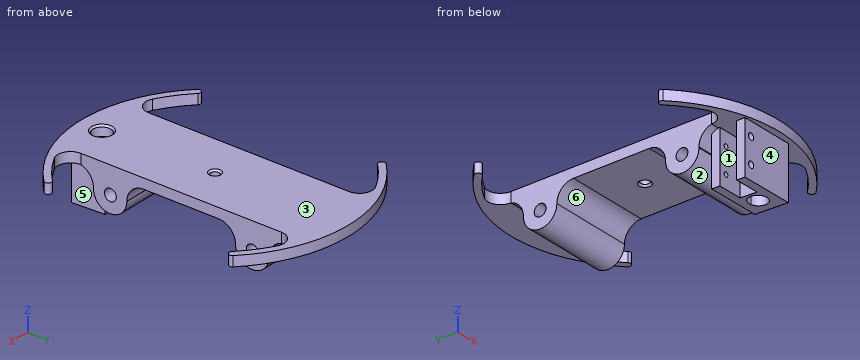
from build123d import *

# Parameters (mm, degrees)
BOSS_EXTRUDE2_DEPTH               = 3.81
BOSS_EXTRUDE4_DEPTH               = 31.75
F_8_CLEARANCE_HOLE1_D             = 4.4958
BOSS_EXTRUDE7_REACH               = 65.711
SKETCH19_R                        = 3.3782
F_1_4_CLEARANCE_HOLE3_D           = 6.7564
F_1_4_CLEARANCE_HOLE3_CSINK_D     = 8.0264
F_1_4_CLEARANCE_HOLE3_CSINK_ANGLE = 90
SKETCH25_R                        = 2.794
CUT_EXTRUDE1_DEPTH                = 3.81
F_2_CLEARANCE_HOLE1_D             = 2.4384
F_2_CLEARANCE_HOLE1_DEPTH         = 3.175
TAP_DRILL_FOR_2_56_TAP1_D         = 1.778
TAP_DRILL_FOR_2_56_TAP1_DEPTH     = 12.7


with BuildPart() as part:
    # Sketch3 → Boss-Extrude2 (new body)
    with BuildSketch(Plane.XY):
        with BuildLine():
            Line((-15.875, -38.1), (-15.875, 38.1))
            ThreePointArc((-15.875, 38.1), (-18.260491841, 42.291797068), (-23.082694008, 42.38179842))
            ThreePointArc((-23.082694008, 42.38179842), (-28.900226452, 38.649767283), (-34.12497326, 34.12497326))
            ThreePointArc((-34.12497326, 34.12497326), (-35.921024484, 34.12497326), (-35.921024484, 35.921024484))
            ThreePointArc((-35.921024484, 35.921024484), (0, 50.8), (35.921024484, 35.921024484))
            ThreePointArc((35.921024484, 35.921024484), (35.921024484, 34.12497326), (34.12497326, 34.12497326))
            ThreePointArc((34.12497326, 34.12497326), (28.900226452, 38.649767283), (23.082694008, 42.38179842))
            ThreePointArc((23.082694008, 42.38179842), (18.260491841, 42.291797068), (15.875, 38.1))
            Line((15.875, 38.1), (15.875, -38.1))
            ThreePointArc((15.875, -38.1), (18.260491841, -42.291797068), (23.082694008, -42.38179842))
            ThreePointArc((23.082694008, -42.38179842), (28.900226452, -38.649767283), (34.12497326, -34.12497326))
            ThreePointArc((34.12497326, -34.12497326), (35.921024484, -34.12497326), (35.921024484, -35.921024484))
            ThreePointArc((35.921024484, -35.921024484), (0, -50.8), (-35.921024484, -35.921024484))
            ThreePointArc((-35.921024484, -35.921024484), (-35.921024484, -34.12497326), (-34.12497326, -34.12497326))
            ThreePointArc((-34.12497326, -34.12497326), (-28.900226452, -38.649767283), (-23.082694008, -42.38179842))
            ThreePointArc((-23.082694008, -42.38179842), (-18.260491841, -42.291797068), (-15.875, -38.1))
        make_face()
    extrude(amount=BOSS_EXTRUDE2_DEPTH)

    # Sketch5 → Boss-Extrude4 (add)
    with BuildSketch(Plane(origin=(15.875, 0, 0), x_dir=(0, 0, -1), z_dir=(1, 0, 0))):
        with BuildLine():
            Line((0, 38.1), (0, 26.99385))
            Line((0, 26.99385), (0, 14.29385))
            ThreePointArc((0, 14.29385), (1.86498297, 18.77886703), (6.35, 20.64385))
            ThreePointArc((6.35, 20.64385), (12.699998494, 26.998224058), (6.341251887, 33.343843974))
            ThreePointArc((6.341251887, 33.343843974), (2.338844583, 34.612930799), (0, 38.1))
        make_face()
        with BuildLine():
            ThreePointArc((6.261703048, -20.644463916), (1.864650947, -18.840779739), (0, -14.469233029))
            Line((0, -14.469233029), (0, -26.99385))
            Line((0, -26.99385), (0, -38.1))
            ThreePointArc((0, -38.1), (2.217611083, -34.670801888), (6.077775616, -33.338012189))
            ThreePointArc((6.077775616, -33.338012189), (6.213919542, -33.33945129), (6.35, -33.34385))
            ThreePointArc((6.35, -33.34385), (12.7, -26.99385), (6.35, -20.64385))
            ThreePointArc((6.35, -20.64385), (6.305852606, -20.644312569), (6.261703048, -20.644463916))
        make_face()
    extrude(amount=-BOSS_EXTRUDE4_DEPTH)

    # #8 Clearance Hole1 (through all)
    with Locations(Plane(origin=(15.875, 0, 0), x_dir=(0, 0, -1), z_dir=(1, 0, 0))):
        with Locations((6.35, 26.99385), (6.35, -26.893399733)):
            Hole(F_8_CLEARANCE_HOLE1_D / 2)

    # Sketch10 → 1/8 (0.125) Diameter Hole1 (revolve, cut)
    with BuildSketch(Plane.YZ):
        Polygon((0, 0), (0, 3.81), (2.2225, 3.81), (1.5875, 3.175), (1.5875, 0.635), (2.2225, 0), align=None)
    revolve(axis=Axis((0, 0, -6.35), (0, 0, 1)), mode=Mode.SUBTRACT)

    # Boss-Extrude7: up to this plane
    boss_extrude7_end = Plane(origin=(-3.551630422, -38.686979812, -19.719207275), z_dir=(0.008390733100517729, 0.03489949670250099, -0.9993556027400597))
    # Sketch19 → Boss-Extrude7 (add, up to the surface)
    with BuildSketch(Plane(origin=(0, 0, 0), x_dir=(-1, 0, 0), z_dir=(0, 0, -1)), mode=Mode.PRIVATE) as boss_extrude7_sk1:
        Polygon((12.7, -38.735), (3.175, -38.735), (3.175, -45.085), (12.7, -45.085), (12.7, -48.26), (-7.62, -48.26), (-7.62, -35.56), (12.7, -35.56), align=None)
        with Locations(Location((-1.27, -41.91, 0), (0, 0, 103.518789087))):
            Circle(SKETCH19_R, mode=Mode.SUBTRACT)
    boss_extrude7_tool1 = split(extrude(boss_extrude7_sk1.sketch, amount=BOSS_EXTRUDE7_REACH, mode=Mode.PRIVATE), bisect_by=boss_extrude7_end, keep=Keep.BOTH, mode=Mode.PRIVATE)
    add(boss_extrude7_tool1.solids().sort_by_distance((-7.9375, -38.495377, 0))[0])

    # 1/4 Clearance Hole3 (through all)
    with Locations(Plane.XY.offset(3.81)):
        with Locations((1.27, -41.91)):
            CounterSinkHole(F_1_4_CLEARANCE_HOLE3_D / 2, F_1_4_CLEARANCE_HOLE3_CSINK_D / 2, counter_sink_angle=F_1_4_CLEARANCE_HOLE3_CSINK_ANGLE)

    # Sketch25 → Cut-Extrude1 (cut)
    with BuildSketch(Plane.ZY.offset(3.175)):
        with Locations(Location((-7.62, -41.91, 0), (0, 0, 270))):
            Circle(SKETCH25_R)
    extrude(amount=-CUT_EXTRUDE1_DEPTH, mode=Mode.SUBTRACT)

    # #2 Clearance Hole1
    with Locations(Plane(origin=(0, -48.26, 0), x_dir=(-1, 0, 0), z_dir=(0, -1, 0))):
        with Locations((9.825, 14.7), (9.825, 5.2)):
            Hole(F_2_CLEARANCE_HOLE1_D / 2, depth=F_2_CLEARANCE_HOLE1_DEPTH)

    # Tap Drill for #2-56 Tap1
    with Locations(Plane(origin=(0, -48.26, 0), x_dir=(-1, 0, 0), z_dir=(0, -1, 0))):
        with Locations((9.825, 14.7), (9.825, 5.2)):
            Hole(TAP_DRILL_FOR_2_56_TAP1_D / 2, depth=TAP_DRILL_FOR_2_56_TAP1_DEPTH)


solid = part.part
Source: CAD feature listing. Evaluate the final solid. Frame: model axes, mm. Face numbers are marked on the shaded views. A direction names the side the tool comes from. Give positions to 0.01 mm unless a question says otherwise; leave off trailing zeros. Write each loop counter-clockwise with the first axis right and the second up, starting at its lowest first coordinate (ties: lowest second). Pieces come first, ordered by that corner, then holes. Notation, with made-up numbers: M -8.5,88.5 L 4.5,88.5 A23 ccw 4.5,100.5 Z; hole C 44,25.25 d10. An arc over 180 degrees is marked long. Return JSON: item names as keys, results as strings. Group by question number.
1) Ray query, L1, parallel to Y at x = 1.5, z = -6.35; L2, parallel to Y at x = -0.5, z = 1; L3, parallel to X at y = -38, z = -14.7. Return the intervals inside material, ascending.
2) Cut plane A-A, the plane y = 37. Output: boundary loops of the cut face in (x, z) (3 decimals).
3) Cut plane B-B, the plane y = 9.5. Output: boundary loops of the cut face in (x, z) (3 decimals).
4) Draft query along Y for the marked faces 1, 2, 3 and 4. Return one class per face: released by +Y, released by -Y, zero draft, split by the parting line, or undercut.
5) Set-up query: the marked faces 5 and 6. Return all of +Z, -Z, +X, -X, +Y, -Y with unobstructed straight access to the full face (end or side cutting, diameter ignored); none if empty.
6) First-contact query: pin 1 Ø10 at (y, z) = (0, -5.5) entering from +X; pin 2 Ø1.5 at (x, z) = (7.5, -16) entering from +Y; pin 3 Ø1.9 at (y, z) = (-43, -7) entering from -X; pin 4 Ø12 at (y, z) = (-3, -4.5) entering from -X (3 decimals). Flat tips, straight axial feed; report the tip coordinate or a pass-through.
Data:
{
 "1": {"L1": "y = -48.26 to -45.28, -38.54 to -35.56, -33.34 to -29.14, -24.65 to -20.64, 20.64 to 24.75, 29.24 to 33.34", "L2": "y = -50.8 to -44.79, -39.03 to -1.51, 1.51 to 50.8", "L3": "x = -12.7 to -10.71, -8.94 to 7.62"},
 "2": {"outline": "M -34.809,0 L -30.984,0 L -30.984,3.81 L -34.809,3.81 Z; M -15.875,-0.397 L 15.875,-0.397 L 15.875,3.81 L -15.875,3.81 Z; M 30.984,0 L 34.809,0 L 34.809,3.81 L 30.984,3.81 Z"},
 "3": {"outline": "M -15.875,0 L 15.875,0 L 15.875,3.81 L -15.875,3.81 Z"},
 "4": {"face 1": "undercut", "face 2": "undercut", "face 3": "zero draft", "face 4": "released by -Y"},
 "5": {"face 5": "-Z, +X, -Y", "face 6": "-Z, +X, -X"},
 "6": {"pin 1": "passes through", "pin 2": "stops at y = -35.56", "pin 3": "stops at x = 3.96", "pin 4": "stops at x = -15.875"}
}
